from build123d import *

# Parameters (mm, degrees)
MAIN_BODY_DEPTH   = 5
SCREW_HOLES_REACH = 18.771


with BuildPart() as part:
    # Schizzo1 → Main body (new, symmetric)
    with BuildSketch(Plane.XY):
        with BuildLine():
            Line((-12.5, -5), (12.5, -5))
            Line((12.5, -5), (12.5, 5))
            Line((12.5, 5), (4.092370951, 5))
            ThreePointArc((4.092370951, 5), (0, 1.15), (-4.092370951, 5))
            Line((-4.092370951, 5), (-12.5, 5))
            Line((-12.5, 5), (-12.5, -5))
        make_face()
    extrude(amount=MAIN_BODY_DEPTH, both=True)

    # Schizzo2 → screw holes (cut, up to next)
    with BuildSketch(Plane.XZ.offset(5), mode=Mode.PRIVATE) as screw_holes_sk1:
        with BuildLine():
            Line((-6.960769515, 1.8), (-6.441154273, 0.9))
            ThreePointArc((-6.441154273, 0.9), (-8, -1.8), (-9.558845727, 0.9))
            Line((-9.558845727, 0.9), (-9.039230485, 1.8))
            Line((-9.039230485, 1.8), (-6.960769515, 1.8))
        make_face()
    screw_holes_tool1 = extrude(screw_holes_sk1.sketch, amount=-SCREW_HOLES_REACH, mode=Mode.PRIVATE) & part.part
    # Schizzo2 → screw holes (cut, up to next)
    with BuildSketch(Plane.XZ.offset(5), mode=Mode.PRIVATE) as screw_holes_sk2:
        with BuildLine():
            Line((6.960769515, 1.8), (9.039230485, 1.8))
            Line((9.039230485, 1.8), (9.558845727, 0.9))
            ThreePointArc((9.558845727, 0.9), (8, -1.8), (6.441154273, 0.9))
            Line((6.441154273, 0.9), (6.960769515, 1.8))
        make_face()
    screw_holes_tool2 = extrude(screw_holes_sk2.sketch, amount=-SCREW_HOLES_REACH, mode=Mode.PRIVATE) & part.part
    add(screw_holes_tool1.solids().sort_by_distance((-8, -5, 0.053309))[0], mode=Mode.SUBTRACT)
    add(screw_holes_tool2.solids().sort_by_distance((8, -5, 0.053309))[0], mode=Mode.SUBTRACT)


solid = part.part
Geometry: final body of the model. Coordinates: model frame, mm. A direction names the side the tool comes from. Give positions to 0.01 mm unless a question says otherwise; leave off trailing zeros. Write each loop counter-clockwise with the first axis right and the second up, starting at its lowest first coordinate (ties: lowest second). Pieces come first, ordered by that corner, then holes. Notation, with made-up numbers: M 71.25,49.25 L 119.25,49.25 A26 ccw 119.25,72.25 Z; hole C 60,-27.75 d3. An arc over 180 degrees is marked long. Answer in a Markdown table with one row per item. Add a question column.
(1) Mould query, pull axis Z, two halves, no side actions, for faces 3 (the cylindrical face through (0.09, 1.15, 0.07)), 4 (the cylindrical face through (8.05, -0.07, -1.8)), 5 (the flat face through (0, 0, 5)). Classes: +Z half, -Z half, draft (parallel to the pull), parting line (faces both ways), or undercut.
(2) Reachability of faces 1 (the flat face through (9.295, -0.07, 1.356)), 2 (the flat face through (-10, 5, 0)) from +Z, -Z, +X, -X, +Y, -Y: full face, straight path, thin tool, end or side. Return the list, or none.
(3) First-contact query: pin 1 (4 mm diameter, centred on x = 8, z = 0, fed in from +Y). Flat tip, straight axial feed; report the tip coordinate or a pass-through.
(4) Section A-A on x = -8. Return loops of the section in (y, z), and give its area (3 significant figures).
(5) Ray query, line 1 (X direction, y = 0.5, z = 0); line 2 (Z direction, x = 8, y = -1.25); line 3 (X direction, y = 0, z = 0.5). Return the intervals inside material, ascending.
(6) Section B-B on y = 3. Return loops of the section in (x, z).
(7) Section C-C on z = 0. Return loops of the section in (x, y), and give its area (3 significant figures).
(8) Section D-D on z = 4. Return loops of the section in (x, y), and give its area (3 significant figures).
Result set:
| question | item | result |
|---|---|---|
| 1 | face 3 | draft |
| 1 | face 4 | undercut |
| 1 | face 5 | +Z half |
| 2 | face 1 | +Y, -Y |
| 2 | face 2 | +Z, -Z, +X, -X, +Y |
| 3 | pin 1 | stops at y = 5 |
| 4 | outline | M -5,-5 L 5,-5 L 5,-1.8 L -5,-1.8 Z; M -5,1.8 L 5,1.8 L 5,5 L -5,5 Z |
| 4 | area | 64.0 mm^2 |
| 5 | line 1 | x = -12.5 to -9.8, -6.2 to 6.2, 9.8 to 12.5 |
| 5 | line 2 | z = -5 to -1.8, 1.8 to 5 |
| 5 | line 3 | x = -12.5 to -9.73, -6.27 to 6.27, 9.73 to 12.5 |
| 6 | outline | M -12.5,-5 L -3.43,-5 L -3.43,5 L -12.5,5 Z; M 3.43,-5 L 12.5,-5 L 12.5,5 L 3.43,5 Z; hole M -9.56,0.9 A1.8 ccw long -6.44,0.9 L -6.96,1.8 L -9.04,1.8 Z; hole M 6.44,0.9 A1.8 ccw long 9.56,0.9 L 9.04,1.8 L 6.96,1.8 Z |
| 7 | outline | M -12.5,-5 L -9.8,-5 L -9.8,5 L -12.5,5 Z; M -6.2,-5 L 6.2,-5 L 6.2,5 L 4.09,5 A4.1 cw -4.09,5 L -6.2,5 Z; M 9.8,-5 L 12.5,-5 L 12.5,5 L 9.8,5 Z |
| 7 | area | 154 mm^2 |
| 8 | outline | M -12.5,-5 L 12.5,-5 L 12.5,5 L 4.09,5 A4.1 cw -4.09,5 L -12.5,5 Z |
| 8 | area | 226 mm^2 |
